Verification items for the finished model (mm, model axes). Coordinates: 2 decimals unless noted, no trailing zeros. Order: outer loops, then holes, each group sorted by start corner. A loop starts at its lowest first (then second) coordinate and runs counter-clockwise, first axis right, second up. Notation, with made-up numbers: M 18.25,53 L 28.25,53 A10 cw 28.25,61 Z; hole C -6,75.5 d11. An arc over 180 degrees is marked long. Return JSON: item names as keys, results as strings. Group by question number.
Q1. Section check A-A, the plane y = 1.05. Count the separate pieces of the cut face and the enclosed holes in it, then the cut area to 3 significant figures.
Q2. Thickness scan on probe 1 along X at (y, z) = (1.5, -5); probe 2 along X at (y, z) = (0.7, -64); probe 3 along Z at (x, y) = (22.5, 1.15). Record the ranges inside material, lowest first.
Q3. Section check C-C, the plane z = -28. Enter the section's corners in (x, y).
Q4. Section check B-B, the plane z = -44. Enter the section's corners in (x, y).
Q5. Go/stop test with flat-tipped pins: pin 1 Ø0.6 at (x, y) = (14, 1) entering from +Z; pin 2 Ø0.6 at (y, z) = (0.5, -2.5) entering from +X. Record where each tip stops, or that it passes through.
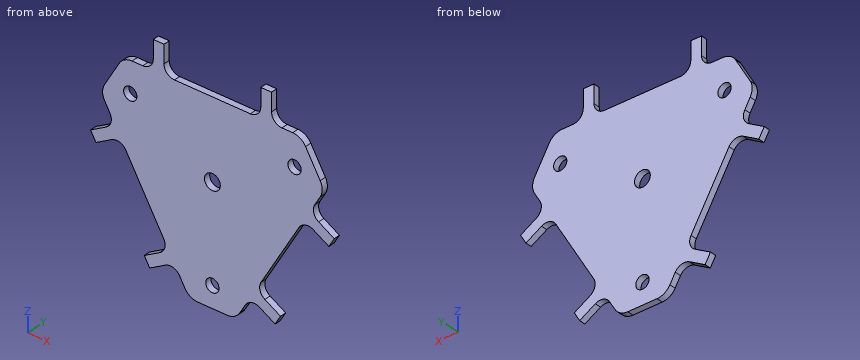
from build123d import *

# Parameters (mm, degrees)
BOSS_EXTRUDE1_DEPTH = 2
SKETCH4_R           = 2.1
CUT_EXTRUDE1_DEPTH  = 105.611811864
SKETCH5_R           = 2.5
CUT_EXTRUDE2_DEPTH  = 105.611811864


with BuildPart() as part:
    # Sketch1 → Boss-Extrude1 (new body)
    with BuildSketch(Plane(origin=(0, 0, 0), x_dir=(1, 0, 0), z_dir=(0, 1, 0))):
        with BuildLine():
            Line((49.096295698, 65.225835767), (47.394589776, 68.173276884))
            ThreePointArc((47.394589776, 68.173276884), (45.674270378, 69.893596282), (43.324270378, 70.523276884))
            Line((43.324270378, 70.523276884), (34.086666071, 70.523276884))
            ThreePointArc((34.086666071, 70.523276884), (31.736666071, 69.893596282), (30.016346673, 68.173276884))
            Line((30.016346673, 68.173276884), (28.314640751, 65.225835767))
            ThreePointArc((28.314640751, 65.225835767), (26.310859767, 63.688280541), (23.806756919, 64.017951935))
            Line((23.806756919, 64.017951935), (18.870412117, 66.867951935))
            Line((18.870412117, 66.867951935), (17.170412117, 63.923465562))
            Line((17.170412117, 63.923465562), (22.106756919, 61.073465562))
            ThreePointArc((22.106756919, 61.073465562), (23.644312145, 59.069684578), (23.314640751, 56.565581729))
            Line((23.314640751, 56.565581729), (11.314640751, 35.780972039))
            ThreePointArc((11.314640751, 35.780972039), (9.310859767, 34.243416812), (6.806756919, 34.573088206))
            Line((6.806756919, 34.573088206), (1.870412117, 37.423088206))
            Line((1.870412117, 37.423088206), (0.170412117, 34.478601833))
            Line((0.170412117, 34.478601833), (5.106756919, 31.628601833))
            ThreePointArc((5.106756919, 31.628601833), (6.644312145, 29.62482085), (6.314640751, 27.120718001))
            Line((6.314640751, 27.120718001), (4.612934829, 24.173276884))
            ThreePointArc((4.612934829, 24.173276884), (3.983254227, 21.823276884), (4.612934829, 19.473276884))
            Line((4.612934829, 19.473276884), (9.231736982, 11.473276884))
            ThreePointArc((9.231736982, 11.473276884), (10.95205638, 9.752957486), (13.30205638, 9.123276884))
            Line((13.30205638, 9.123276884), (16.705468225, 9.123276884))
            ThreePointArc((16.705468225, 9.123276884), (19.038920602, 8.156729262), (20.005468225, 5.823276884))
            Line((20.005468225, 5.823276884), (20.005468225, 0.123276884))
            Line((20.005468225, 0.123276884), (23.405468225, 0.123276884))
            Line((23.405468225, 0.123276884), (23.405468225, 5.823276884))
            ThreePointArc((23.405468225, 5.823276884), (24.372015847, 8.156729262), (26.705468225, 9.123276884))
            Line((26.705468225, 9.123276884), (50.705468225, 9.123276884))
            ThreePointArc((50.705468225, 9.123276884), (53.038920602, 8.156729262), (54.005468225, 5.823276884))
            Line((54.005468225, 5.823276884), (54.005468225, 0.123276884))
            Line((54.005468225, 0.123276884), (57.405468225, 0.123276884))
            Line((57.405468225, 0.123276884), (57.405468225, 5.823276884))
            ThreePointArc((57.405468225, 5.823276884), (58.372015847, 8.156729262), (60.705468225, 9.123276884))
            Line((60.705468225, 9.123276884), (64.108880069, 9.123276884))
            ThreePointArc((64.108880069, 9.123276884), (66.458880069, 9.752957486), (68.179199467, 11.473276884))
            Line((68.179199467, 11.473276884), (72.79800162, 19.473276884))
            ThreePointArc((72.79800162, 19.473276884), (73.427682222, 21.823276884), (72.79800162, 24.173276884))
            Line((72.79800162, 24.173276884), (71.096295698, 27.120718001))
            ThreePointArc((71.096295698, 27.120718001), (70.766624304, 29.62482085), (72.304179531, 31.628601833))
            Line((72.304179531, 31.628601833), (77.240524332, 34.478601833))
            Line((77.240524332, 34.478601833), (75.540524332, 37.423088206))
            Line((75.540524332, 37.423088206), (70.604179531, 34.573088206))
            ThreePointArc((70.604179531, 34.573088206), (68.100076682, 34.243416812), (66.096295698, 35.780972039))
            Line((66.096295698, 35.780972039), (54.096295698, 56.565581729))
            ThreePointArc((54.096295698, 56.565581729), (53.766624304, 59.069684578), (55.304179531, 61.073465562))
            Line((55.304179531, 61.073465562), (60.240524332, 63.923465562))
            Line((60.240524332, 63.923465562), (58.540524332, 66.867951935))
            Line((58.540524332, 66.867951935), (53.604179531, 64.017951935))
            ThreePointArc((53.604179531, 64.017951935), (51.100076682, 63.688280541), (49.096295698, 65.225835767))
        make_face()
    extrude(amount=BOSS_EXTRUDE1_DEPTH)

    # Sketch4 → Cut-Extrude1 (cut, through all)
    with BuildSketch(Plane(origin=(0, 2, 0), x_dir=(1, 0, 0), z_dir=(0, 1, 0))):
        with Locations(Location((38.705468225, 63.823276884, 0), (0, 0, 270))):
            Circle(SKETCH4_R)
        with Locations(Location((12.724706111, 18.823276884, 0), (0, 0, 270))):
            Circle(SKETCH4_R)
        with Locations(Location((64.686230338, 18.823276884, 0), (0, 0, 270))):
            Circle(SKETCH4_R)
    extrude(amount=-CUT_EXTRUDE1_DEPTH, mode=Mode.SUBTRACT)

    # Sketch5 → Cut-Extrude2 (cut, through all)
    with BuildSketch(Plane(origin=(0, 2, 0), x_dir=(1, 0, 0), z_dir=(0, 1, 0))):
        with Locations(Location((38.705468225, 33.823276884, 0), (0, 0, 270))):
            Circle(SKETCH5_R)
    extrude(amount=-CUT_EXTRUDE2_DEPTH, mode=Mode.SUBTRACT)


solid = part.part
Numbers:
{
 "1": {"separate pieces": "1", "enclosed holes": "4", "area": "3,030 mm2"},
 "2": {"probe 1": "x = 20.01 to 23.41, 54.01 to 57.41", "probe 2": "x = 17.21 to 23.84, 27.08 to 36.61, 40.8 to 50.34, 53.57 to 60.2", "probe 3": "z = -64.77 to -60.81, -55.15 to -0.12"},
 "3": {"outline": "M 6.67,0 L 70.75,0 L 70.75,2 L 6.67,2 Z"},
 "4": {"outline": "M 16.06,0 L 61.35,0 L 61.35,2 L 16.06,2 Z"},
 "5": {"pin 1": "stops at z = -9.12", "pin 2": "stops at x = 57.41"}
}
